Autodesk Inventor part; units mm, degrees
ref_plane "YZ Plane" through (0, 0, 0) normal (1, 0, 0) x (0, 1, 0)
ref_plane "XZ Plane" through (0, 0, 0) normal (0, 1, 0) x (-1, 0, 0)
ref_plane "XY Plane" through (0, 0, 0) normal (0, 0, 1) x (1, 0, 0)
sketch "Sketch1" plane through (0, 0, 0) normal (0, 1, 0) x (-1, 0, 0)
  circle A0 centre (0, 0) radius 57.15
  circle A1 centre (0, 0) radius 44.5
  dimension "d0" = 114.3
  dimension "d1" = 89
extrude "Extrusion1" add sketch "Sketch1" along normal blind 10
sketch "Sketch3" plane through (0, 10, 0) normal (0, 1, 0) x (1, 0, 0)
  line L0 (0, 0) -> (0, -50.4952)
  point P0 (50.4952, 0)
  point P1 (50.4952, 0)
  point P2 (0, 50.4952)
  point P3 (0, 50.4952)
  point P4 (-50.4952, 0)
  point P5 (-50.4952, 0)
  dimension "d18" = 50.4952
  dimension "d21" = 360
hole "Hole1" at (0, 10, 50.4952) at (50.4952, 10, 0) at (0, 10, -50.4952) at (-50.4952, 10, 0) direction (0, -1, 0) diameter 5.7 depth 15.6718 tip angle 118 countersink diameter 9.525 countersink angle 82
properties part number "innerbearingwheel"
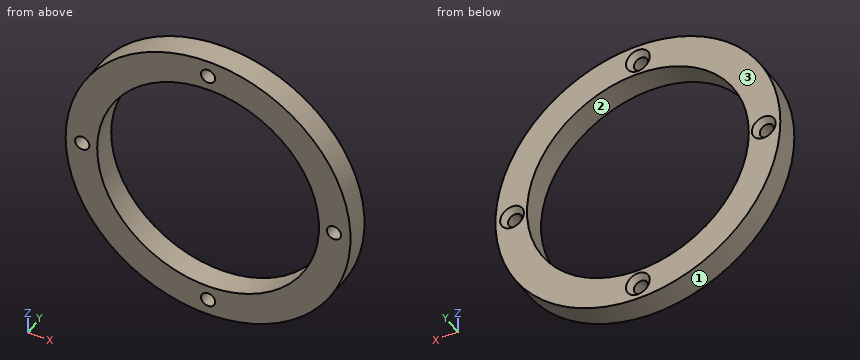
Verification items for the finished model (mm, model axes). Face numbers are marked on the shaded views. Give positions to 0.01 mm unless a question says otherwise; leave off trailing zeros. Order: outer loops, then holes, each group sorted by start corner. A loop starts at its lowest first (then second) coordinate and runs counter-clockwise, first axis right, second up. Notation, with made-up numbers: (57.5, 88) -> (109.5, 88) arc R19 cw to (109.5, 93) -> close; hole circle Ø10 at (40, 45.5). An arc over 180 degrees is marked (long way). One line per item, written item: value.
(1) Sectioned sample at D-D on z = -13. Record the cut outline in (x, y), then the cut area to 3 significant figures.
Final values:
outline: (-55.65, 0) -> (-42.56, 0) -> (-42.56, 10) -> (-55.65, 10) -> close; (42.56, 0) -> (55.65, 0) -> (55.65, 10) -> (42.56, 10) -> close
area: 262 mm^2
(2) Sectioned sample at B-B on x = 0. Record the cut outline in (y, z), then the cut area to 3 significant figures.
Final values:
outline: (0, -57.15) -> (10, -57.15) -> (10, -55.26) -> (7.8, -53.35) -> (0, -53.35) -> close; (0, -47.65) -> (7.8, -47.65) -> (10, -45.73) -> (10, -44.5) -> (0, -44.5) -> close; (0, 44.5) -> (10, 44.5) -> (10, 45.73) -> (7.8, 47.65) -> (0, 47.65) -> close; (0, 53.35) -> (7.8, 53.35) -> (10, 55.26) -> (10, 57.15) -> (0, 57.15) -> close
area: 131 mm^2
(3) Gauge pin test, flat ends, axial feed: pin 1 (5 mm diameter, centred on y = 2, z = -10.5, fed in from +X); pin 2 (4.5 mm diameter, centred on x = -50.5, z = 0, fed in from -Y); pin 3 (7.5 mm diameter, centred on x = 0, z = -50.5, fed in from +Y); pin 4 (5 mm diameter, centred on x = 3.5, y = 6.5, fed in from +Z). Record the tip position at first contact, or that the pin passes through.
Final values:
pin 1: x = 56.59
pin 2: through
pin 3: y = 8.84
pin 4: z = 57.14
(4) Sectioned sample at A-A on z = 0. Record the cut outline in (x, y), then the cut area to 3 significant figures.
Final values:
outline: (-57.15, 0) -> (-53.35, 0) -> (-53.35, 7.8) -> (-55.26, 10) -> (-57.15, 10) -> close; (-47.65, 0) -> (-44.5, 0) -> (-44.5, 10) -> (-45.73, 10) -> (-47.65, 7.8) -> close; (44.5, 0) -> (47.65, 0) -> (47.65, 7.8) -> (45.73, 10) -> (44.5, 10) -> close; (53.35, 0) -> (57.15, 0) -> (57.15, 10) -> (55.26, 10) -> (53.35, 7.8) -> close
area: 131 mm^2
(5) Draft check along Z on the marked faces 1, 2 and 3. Enter one of: pulls with the +Z half, pulls with the -Z half, needs draft (parallel to the pull), parting line crosses it, or undercut.
Final values:
face 1: parting line crosses it
face 2: undercut
face 3: needs draft
(6) Scan lines: line 1 along Z through (x, y) = (0, 5.75); line 2 along X through (y, z) = (9.5, -2.5); line 3 along Z through (x, y) = (0.5, 1.5). Record each from-to range of solid material in increasing order. Write a range as [from, to].
Final values:
line 1: [-57.15, -53.35], [-47.65, -44.5], [44.5, 47.65], [53.35, 57.15]
line 2: [-57.1, -54.03], [-46.96, -44.43], [44.43, 46.96], [54.03, 57.1]
line 3: [-57.15, -53.3], [-47.69, -44.5], [44.5, 47.69], [53.3, 57.15]
(7) Sectioned sample at C-C on x = 21. Record the cut outline in (y, z).
Final values:
outline: (0, -53.15) -> (10, -53.15) -> (10, -39.23) -> (0, -39.23) -> close; (0, 39.23) -> (10, 39.23) -> (10, 53.15) -> (0, 53.15) -> close
